The listing builds one solid part. Answer for the finished solid, in the listing's coordinates (mm). A direction names the side the tool comes from. Coordinates: 2 decimals unless noted, no trailing zeros. Order: outer loops, then holes, each group sorted by start corner. A loop starts at its lowest first (then second) coordinate and runs counter-clockwise, first axis right, second up. Notation, with made-up numbers: (81.5, 54.5) -> (112.5, 54.5) arc R20 cw to (112.5, 62.5) -> close; hole circle Ø1 at (25, 12). An arc over 180 degrees is marked (long way). One line per question, with ' | ' between items.
from build123d import *

# Parameters (mm, degrees)
F1_DEPTH   = 22.606
F2_R       = 5.08
F5_D       = 12.7
F5_ON_F4_D = 12.7


with BuildPart() as f1:
    # F0 (on Top) → F1 (new body)
    with BuildSketch(Plane.XY):
        with BuildLine():
            ThreePointArc((0, -74.1540131918), (27.9531270487, -68.6836251274), (51.7820146668, -53.0795688518))
            Line((51.7820146668, -53.0795688518), (0, 0))
            Line((0, 0), (0, -74.1540131918))
        make_face()
        with BuildLine():
            ThreePointArc((51.7820146668, -53.0795688518), (68.3325027755, -28.8008113926), (74.1540131918, 0))
            Line((74.1540131918, 0), (0, 0))
            Line((0, 0), (51.7820146668, -53.0795688518))
        make_face()
        with BuildLine():
            Line((0, 0), (74.1540131918, 0))
            ThreePointArc((74.1540131918, 0), (68.6836251274, 27.9531270487), (53.0795688518, 51.7820146668))
            Line((53.0795688518, 51.7820146668), (0, 0))
        make_face()
        with BuildLine():
            Line((0, 0), (53.0795688518, 51.7820146668))
            ThreePointArc((53.0795688518, 51.7820146668), (28.8008113926, 68.3325027755), (0, 74.1540131918))
            Line((0, 74.1540131918), (0, 0))
        make_face()
        with BuildLine():
            Line((-51.7820146668, 53.0795688518), (0, 0))
            Line((0, 0), (0, 74.1540131918))
            ThreePointArc((0, 74.1540131918), (-27.9531270487, 68.6836251274), (-51.7820146668, 53.0795688518))
        make_face()
        with BuildLine():
            Line((-74.1540131918, 0), (0, 0))
            Line((0, 0), (-51.7820146668, 53.0795688518))
            ThreePointArc((-51.7820146668, 53.0795688518), (-68.3325027755, 28.8008113926), (-74.1540131918, 0))
        make_face()
        with BuildLine():
            Line((-53.0795688518, -51.7820146668), (0, 0))
            Line((0, 0), (-74.1540131918, 0))
            ThreePointArc((-74.1540131918, 0), (-68.6836251274, -27.9531270487), (-53.0795688518, -51.7820146668))
        make_face()
        with BuildLine():
            Line((0, -74.1540131918), (0, 0))
            Line((0, 0), (-53.0795688518, -51.7820146668))
            ThreePointArc((-53.0795688518, -51.7820146668), (-28.8008113926, -68.3325027755), (0, -74.1540131918))
        make_face()
    extrude(amount=F1_DEPTH)

    # F2
    f2_edges = [f1.edges().sort_by_distance(p)[0] for p in [
        (53.079569, 51.782015, 22.606),
        (53.079569, 51.782015, 0),
    ]]
    fillet(f2_edges, radius=F2_R)

    # F5 (through all)
    with Locations(Plane.XY.offset(22.606)):
        with Locations((-18.9406760037, 16.0708744079), (16.8744213879, 15.8412903547), (-18.7110900879, -16.300458461)):
            Hole(F5_D / 2)

    # F5 on F4 (through all)
    with Locations(Plane.XY.offset(22.606)):
        with Locations((18.0223360658, -16.5300425142), (-18.9406760037, 16.300458461)):
            Hole(F5_ON_F4_D / 2)


solid = f1.part
Item 1: Section A-A, the plane z = 12.25 is taken. Give the vertices of the cut face in (x, y).
Computed values:
outline: circle Ø148.31 at (0, 0); hole (-25.29, 16.19) arc R6.35 ccw (long way) to (-12.59, 16.19) arc R6.35 ccw (long way) to start; hole circle Ø12.7 at (-18.71, -16.3); hole circle Ø12.7 at (16.87, 15.84); hole circle Ø12.7 at (18.02, -16.53)
Item 2: For faces 3 (the face through (-1, 1, 22.606)), 4 (the face through (-19.08, 22.65, 11.14)), determine the directions among +Z, -Z, +X, -X, +Y, -Y from which every point of the face is accessible in a straight line to the end or side of a thin tool.
Computed values:
face 3: +Z, +X, -X, +Y, -Y | face 4: +Z, -Z
Item 3: Determine the mould class of faces 1 (the face through (-1, 1, 0)), 2 (the face through (23.061, -20.394, 11.145)) for opening direction Y: pulls with the +Y half, pulls with the -Y half, needs draft (parallel to the pull), parting line crosses it, or undercut.
Computed values:
face 1: needs draft | face 2: undercut
Item 4: Section B-B, the plane x = 18.5 is taken. Count the separate pieces of the cut face and the enclosed holes in it, plus the area to 3 significant figures.
Computed values:
separate pieces: 3 | enclosed holes: 0 | area: 2,660 mm^2
Item 5: Each of these flat-tipped pins is pushed along its axis until it touches: pin 1 Ø4 at (y, z) = (6, 8) entering from -X; pin 2 Ø4 at (x, z) = (25, 17.5) entering from -Y; pin 3 Ø8 at (y, z) = (-11, 9.5) entering from +X; pin 4 Ø1.5 at (x, z) = (-0.5, 7) entering from +Y. Where does it stop, or does it pass through?
Computed values:
pin 1: stops at x = -74.05 | pin 2: stops at y = -70.5 | pin 3: stops at x = 73.82 | pin 4: stops at y = 74.15
Item 6: Find the intervals of material crossed by L1, parallel to Y at x = -18, z = 21.75; L2, parallel to X at y = -13, z = 8; L3, parallel to Z at x = -67, y = -17.5, in increasing order.
Computed values:
L1: y = -69.61 to -22.61, -9.99 to 9.79, 22.58 to 69.61 | L2: x = -73.01 to -24.14, -13.29 to 12.74, 23.3 to 73.01 | L3: z = 0 to 22.6
